The model under review builds one solid part; all positions refer to its coordinate system, in mm. Face numbers are marked on the shaded views. A direction names the side the tool comes from. Coordinates: 2 decimals unless noted, no trailing zeros. Loops run counter-clockwise (first coordinate to the right, second up) from the corner with the lowest first, then second, coordinate; pieces in that order, holes last. Notation, with made-up numbers: (9.25, 3) - (14.25, 3) arc R24 ccw to (14.25, 17) - close; hole circle Ø10 at (34.5, 45). An arc over 180 degrees is marked (long way). Use a Markdown table: item, result. Add a question column.
1) To check wall thickness, follow L1, parallel to Z at x = 0, y = 4; L2, parallel to Y at x = 3.5, z = 5.25; L3, parallel to X at y = 5.75, z = 3. State the ranges of each line that lie inside material, in increasing order. Write a range as [from, to].
2) Add section A-A, the plane z = 0. Give the boundary of the cut face in (x, y).
3) For the marked faces 1 and 2, list the 3-axis set-ups (+Z, -Z, +X, -X, +Y, -Y) from which the entire face can be reached by the end or side of a thin tool; tool diameter is ignored.
4) Add section D-D, the plane z = -3.75. Give the boundary of the cut face in (x, y).
5) Add section B-B, the plane x = 0. Give the boundary of the cut face in (y, z).
6) Add section C-C, the plane y = 4. Give the boundary of the cut face in (x, z), and give its area (3 significant figures).
7) The part is to be moulded in two halves that separate along Z. For the marked faces 3, 4 and 5, say which applies: pulls with the +Z half, pulls with the -Z half, needs draft (parallel to the pull), parting line crosses it, or undercut.
8) Clearance check with flat-ended pins moving along their axes: pin 1 (3 mm diameter, centred on x = 5, y = 0, fed in from +Z); pin 2 (1 mm diameter, centred on x = 1, y = 3.5, fed in from -Z); pin 3 (3 mm diameter, centred on x = 2.5, y = 6.5, fed in from -Z). State where each tip first meets the part, or that it passes through.
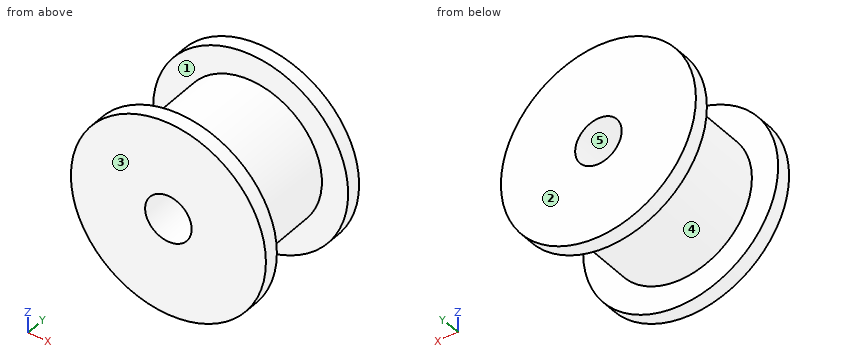
Autodesk Inventor part; units mm, degrees
ref_plane "YZ Plane" through (0, 0, 0) normal (1, 0, 0) x (0, 1, 0)
ref_plane "XZ Plane" through (0, 0, 0) normal (0, 1, 0) x (-1, 0, 0)
ref_plane "XY Plane" through (0, 0, 0) normal (0, 0, 1) x (1, 0, 0)
sketch "Boceto1" plane through (0, 0, 0) normal (0, 1, 0) x (-1, 0, 0)
  circle A0 centre (0, 0) radius 4.75
  dimension "d0" = 9.5
extrude "Extrusión1" add sketch "Boceto1" along normal blind 6.5
sketch "Boceto2" plane through (0, 6.5, 0) normal (0, 1, 0) x (1, 0, 0)
  circle A0 centre (0, 0) radius 4.75
  circle A1 centre (0, 0) radius 6.5
  dimension "d3" = 13
extrude "Extrusión2" add sketch "Boceto2" along normal blind 1 contours A0 | A1
sketch "Boceto3" plane through (0, 0, 0) normal (0, -1, 0) x (1, 0, 0)
  circle A0 centre (0, 0) radius 6.5
extrude "Extrusión3" add sketch "Boceto3" along normal blind 1
sketch "Boceto4" plane through (0, -1, 0) normal (0, -1, 0) x (1, 0, 0)
  circle A0 centre (0, 0) radius 1.55
  dimension "d8" = 3.1
extrude "Extrusión4" cut sketch "Boceto4" against normal through all
properties part number "Polea Lisa" material "Acero inoxidable"
From the geometry:
| question | item | result |
|---|---|---|
| 1 | L1 | z = [-4.75, -1.55], [1.55, 4.75] |
| 1 | L2 | y = [-1, 0], [6.5, 7.5] |
| 1 | L3 | x = [-3.68, 3.68] |
| 2 | outline | (-6.5, -1) - (-1.55, -1) - (-1.55, 7.5) - (-6.5, 7.5) - (-6.5, 6.5) - (-4.75, 6.5) - (-4.75, 0) - (-6.5, 0) - close; (1.55, -1) - (6.5, -1) - (6.5, 0) - (4.75, 0) - (4.75, 6.5) - (6.5, 6.5) - (6.5, 7.5) - (1.55, 7.5) - close |
| 3 | face 1 | none |
| 3 | face 2 | +Z, -Z, +X, -X, +Y |
| 4 | outline | (-5.31, -1) - (5.31, -1) - (5.31, 0) - (2.92, 0) - (2.92, 6.5) - (5.31, 6.5) - (5.31, 7.5) - (-5.31, 7.5) - (-5.31, 6.5) - (-2.92, 6.5) - (-2.92, 0) - (-5.31, 0) - close |
| 5 | outline | (-1, -6.5) - (0, -6.5) - (0, -4.75) - (6.5, -4.75) - (6.5, -6.5) - (7.5, -6.5) - (7.5, -1.55) - (-1, -1.55) - close; (-1, 1.55) - (7.5, 1.55) - (7.5, 6.5) - (6.5, 6.5) - (6.5, 4.75) - (0, 4.75) - (0, 6.5) - (-1, 6.5) - close |
| 6 | outline | circle Ø9.5 at (0, 0); hole circle Ø3.1 at (0, 0) |
| 6 | area | 63.3 mm^2 |
| 7 | face 3 | needs draft |
| 7 | face 4 | parting line crosses it |
| 7 | face 5 | undercut |
| 8 | pin 1 | stops at z = 5.48 |
| 8 | pin 2 | stops at z = -4.72 |
| 8 | pin 3 | stops at z = -6.42 |
